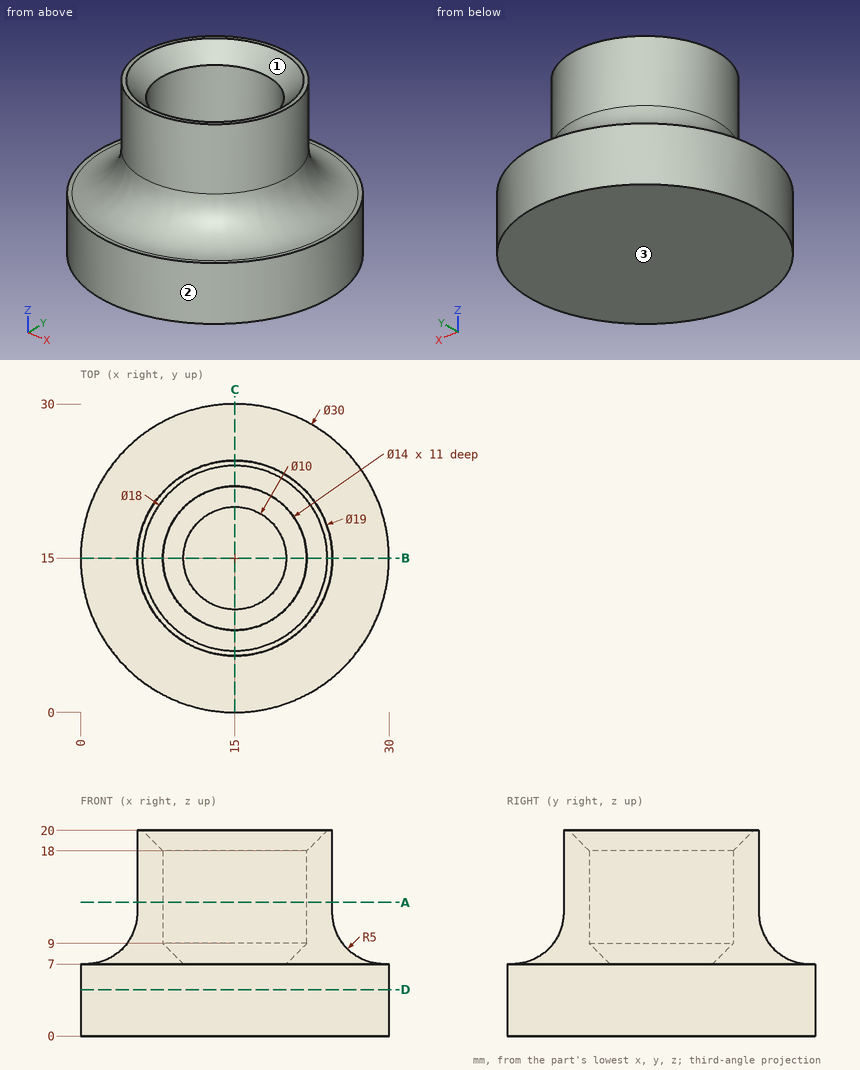
The drawing under review shows one solid part. Ordinate dimensions are in mm from its lowest x, y, z. Round coordinates to 2 decimals unless told otherwise and drop trailing zeros. Write each loop counter-clockwise with the first axis right and the second up, starting at its lowest first coordinate (ties: lowest second). Pieces come first, ordered by that corner, then holes. Notation, with made-up numbers: (52.25, 11.25) - (101.25, 11.25) arc R24 ccw to (101.25, 21.25) - close; hole circle Ø8 at (-40, 26). An arc over 180 degrees is marked (long way). Use a Markdown table: item, result. Add a question column.
1. Clearance check with flat-ended pins moving along their axes: pin 1 (8 mm diameter, centred on y = 23, z = 10, fed in from -X); pin 2 (5 mm diameter, centred on x = 12.5, y = 16.5, fed in from +Z); pin 3 (11 mm diameter, centred on x = 15, y = 15, fed in from +Z); pin 4 (10 mm diameter, centred on y = 10.5, z = 9, fed in from +X). State where each tip first meets the part, or that it passes through.
2. Mouldability with a two-part tool opening along Y and no side actions: class the marked faces 1, 2 and 3 as +Y half, -Y half, draft (parallel to the pull), parting line (faces both ways), or undercut.
3. We need section D-D (z = 4.5). State the section outline as (x, y) points.
4. We need section A-A (z = 13). State the section outline as (x, y) points.
5. We need section B-B (y = 15). State the section outline as (x, z) points, then the cut area to 3 significant figures.
6. Wall thickness on probe 1 along Y at (x, z) = (15, 13.25); probe 2 along Z at (x, y) = (11, 17): over which ranges is each line inside the solid? List them lowest first.
Output:
| question | item | result |
|---|---|---|
| 1 | pin 1 | stops at x = 0.99 |
| 1 | pin 2 | stops at z = 7.42 |
| 1 | pin 3 | stops at z = 7.5 |
| 1 | pin 4 | stops at x = 30 |
| 2 | face 1 | undercut |
| 2 | face 2 | parting line |
| 2 | face 3 | draft |
| 3 | outline | circle Ø30 at (15, 15) |
| 4 | outline | circle Ø19 at (15, 15); hole circle Ø14 at (15, 15) |
| 5 | outline | (0, 0) - (30, 0) - (30, 7) - (29.5, 7) arc R5 cw to (24.5, 12) - (24.5, 20) - (24, 20) - (22, 18) - (22, 9) - (20, 7) - (10, 7) - (8, 9) - (8, 18) - (6, 20) - (5.5, 20) - (5.5, 12) arc R5 cw to (0.5, 7) - (0, 7) - close |
| 5 | area | 286 mm2 |
| 6 | probe 1 | y = 5.5 to 8, 22 to 24.5 |
| 6 | probe 2 | z = 0 to 7 |
